from build123d import *

# Parameters (mm, degrees)
SKETCH1_R           = 75
BOSS_EXTRUDE1_DEPTH = 5
SKETCH2_W           = 50
SKETCH2_H           = 20
BOSS_EXTRUDE2_DEPTH = 20
CUT_EXTRUDE1_START  = -2.5
CUT_EXTRUDE1_DEPTH  = 18
CUT_EXTRUDE2_DEPTH  = 27
CUT_EXTRUDE3_REACH  = 115.275
CUT_EXTRUDE4_REACH  = 117.109
SKETCH6_R           = 1


with BuildPart() as part:
    # Sketch1 → Boss-Extrude1 (new body)
    with BuildSketch(Plane(origin=(0, 0, 0), x_dir=(1, 0, 0), z_dir=(0, 1, 0))):
        with Locations(Location((0, 0, 0), (0, 0, 270))):
            Circle(SKETCH1_R)
    extrude(amount=BOSS_EXTRUDE1_DEPTH)

    # Sketch2 → Boss-Extrude2 (add)
    with BuildSketch(Plane(origin=(0, 0, 0), x_dir=(-1, 0, 0), z_dir=(0, -1, 0))):
        with Locations((-15, -40)):
            Rectangle(SKETCH2_W, SKETCH2_H)
    extrude(amount=BOSS_EXTRUDE2_DEPTH)

    # Sketch3 → Cut-Extrude1 (cut)
    with BuildSketch(Plane.ZY.offset(10).offset(CUT_EXTRUDE1_START)):
        with BuildLine():
            Line((32, -15), (32, -20))
            Line((32, -20), (48, -20))
            Line((48, -20), (48, -15))
            ThreePointArc((48, -15), (40, -7), (32, -15))
        make_face()
    extrude(amount=-CUT_EXTRUDE1_DEPTH, mode=Mode.SUBTRACT)

    # Sketch4 → Cut-Extrude2 (cut)
    with BuildSketch(Plane.ZY.offset(-10.5)):
        with BuildLine():
            Line((31, -15), (31, -20))
            Line((31, -20), (49, -20))
            Line((49, -20), (49, -15))
            ThreePointArc((49, -15), (40, -6), (31, -15))
        make_face()
    extrude(amount=-CUT_EXTRUDE2_DEPTH, mode=Mode.SUBTRACT)

    # Sketch5 → Cut-Extrude3 (cut, up to next)
    with BuildSketch(Plane(origin=(-7.5, 0, 0), x_dir=(0, 0, -1), z_dir=(1, 0, 0)), mode=Mode.PRIVATE) as cut_extrude3_sk1:
        with BuildLine():
            Line((-36.25, -15), (-36.25, -20))
            Line((-36.25, -20), (-43.75, -20))
            Line((-43.75, -20), (-43.75, -15))
            ThreePointArc((-43.75, -15), (-40, -11.25), (-36.25, -15))
        make_face()
    cut_extrude3_tool1 = extrude(cut_extrude3_sk1.sketch, amount=-CUT_EXTRUDE3_REACH, mode=Mode.PRIVATE) & part.part
    add(cut_extrude3_tool1.solids().sort_by_distance((-7.5, -15.983293, 40))[0], mode=Mode.SUBTRACT)

    # Sketch6 → Cut-Extrude4 (cut, up to next)
    with BuildSketch(Plane.ZY.offset(10), mode=Mode.PRIVATE) as cut_extrude4_sk1:
        with Locations((45.5, -15)):
            Circle(SKETCH6_R)
    cut_extrude4_tool1 = extrude(cut_extrude4_sk1.sketch, amount=-CUT_EXTRUDE4_REACH, mode=Mode.PRIVATE) & part.part
    # Sketch6 → Cut-Extrude4 (cut, up to next)
    with BuildSketch(Plane.ZY.offset(10), mode=Mode.PRIVATE) as cut_extrude4_sk2:
        with Locations((34.5, -15)):
            Circle(SKETCH6_R)
    cut_extrude4_tool2 = extrude(cut_extrude4_sk2.sketch, amount=-CUT_EXTRUDE4_REACH, mode=Mode.PRIVATE) & part.part
    add(cut_extrude4_tool1.solids().sort_by_distance((-10, -15, 45.5))[0], mode=Mode.SUBTRACT)
    add(cut_extrude4_tool2.solids().sort_by_distance((-10, -15, 34.5))[0], mode=Mode.SUBTRACT)


solid = part.part
Design review of the part built by this model. Coordinates are the model's own, in mm. A direction names the side the tool comes from. Round coordinates to 2 decimals unless told otherwise and drop trailing zeros. Loops run counter-clockwise (first coordinate to the right, second up) from the corner with the lowest first, then second, coordinate; pieces in that order, holes last. Notation, with made-up numbers: (-22.5, -25) - (1.5, -25) arc R14 cw to (1.5, -15) - close; hole circle Ø7 at (64.25, 39). An arc over 180 degrees is marked (long way). One line per item, written item: value. Start each with the question number.
1) Consider section A-A on x = 0. Give the boundary of the cut face in (y, z).
2) Insertion check: pin 1 Ø1.2 at (x, y) = (-9.5, -17.5) entering from +Z; pin 2 Ø10 at (x, y) = (26, -15) entering from -Z; pin 3 Ø2.5 at (y, z) = (-15, 45.5) entering from -X. Each pin has a flat end and moves straight along its axis. Give the tip position at first contact, or say it passes through.
3) Consider section B-B on z = 40. Give the boundary of the cut face in (x, y).
4) For faces 4 (the flat face through (1, -17, 32)), 5 (the flat face through (-10, -10, 40)), 6 (the flat face through (40, -10, 40)), list the 3-axis set-ups (+Z, -Z, +X, -X, +Y, -Y) from which the entire face can be reached by the end or side of a thin tool; tool diameter is ignored.
5) Consider section C-C on y = 3. Give the boundary of the cut face in (x, z).
6) To check wall thickness, follow L1, parallel to X at y = -14.25, z = 47; L2, parallel to Y at x = -1, z = 65; L3, parallel to Z at x = -9.5, y = -10.5. State the ranges of each line that lie inside material, in increasing order. Write a range as from..to.
7) Draft analysis for pull direction X (two halves, no side actions). For faces 1 (the flat face through (1, 0, -1)), 2 (the cylindrical face through (-45.636, 2.465, -59.517)), 3 (the flat face through (10.5, -7, 38)), state which applies: +X half, -X half, draft (parallel to the pull), parting line (faces both ways), or undercut.
8) Consider section D-D on x = 26. Give the boundary of the cut face in (y, z), then the cut area to 3 significant figures.
Reported:
1. outline: (-20, 30) - (0, 30) - (0, -75) - (5, -75) - (5, 75) - (0, 75) - (0, 50) - (-20, 50) - (-20, 48) - (-15, 48) arc R8 cw to (-15, 32) - (-20, 32) - close
2. pin 1: stops at z = 50
2. pin 2: stops at z = 30
2. pin 3: stops at x = -10
3. outline: (-63.44, 0) - (-10, 0) - (-10, -11.25) - (-7.5, -11.25) - (-7.5, -7) - (10.5, -7) - (10.5, -6) - (37.5, -6) - (37.5, -20) - (40, -20) - (40, 0) - (63.44, 0) - (63.44, 5) - (-63.44, 5) - close
4. face 4: -Y
4. face 5: +Z, -Z, -X, -Y
4. face 6: +Z, -Z, +X, -Y
5. outline: circle Ø150 at (0, 0)
6. L1: x = -10..-7.5, 37.5..40
6. L2: y = 0..5
6. L3: z = 30..50
7. face 1: draft
7. face 2: parting line
7. face 3: undercut
8. outline: (-20, 30) - (0, 30) - (0, -70.35) - (5, -70.35) - (5, 70.35) - (0, 70.35) - (0, 50) - (-20, 50) - (-20, 49) - (-15, 49) arc R9 cw to (-15, 31) - (-20, 31) - close
8. area: 886 mm^2
